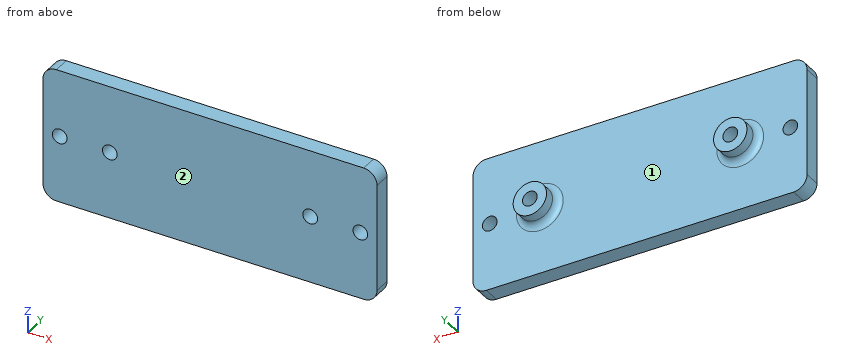
from build123d import *

# Parameters (mm, degrees)
BOSS_EXTRUDE1_DEPTH = 3.175
SKETCH2_R           = 3.175
BOSS_EXTRUDE2_DEPTH = 3.175
SKETCH3_R           = 1.397
CUT_EXTRUDE1_DEPTH  = 7.35
FILLET1_R           = 1.27
CUT_EXTRUDE2_REACH  = 5.175
SKETCH4_R           = 1.397


with BuildPart() as part:
    # Sketch1 → Boss-Extrude1 (new body)
    with BuildSketch(Plane(origin=(0, 0, 0), x_dir=(1, 0, 0), z_dir=(0, 1, 0))):
        with BuildLine():
            Line((-29.21, -12.7), (29.21, -12.7))
            ThreePointArc((29.21, -12.7), (31.006051224, -11.956051224), (31.75, -10.16))
            Line((31.75, -10.16), (31.75, 10.16))
            ThreePointArc((31.75, 10.16), (31.006051224, 11.956051224), (29.21, 12.7))
            Line((29.21, 12.7), (-29.21, 12.7))
            ThreePointArc((-29.21, 12.7), (-31.006051224, 11.956051224), (-31.75, 10.16))
            Line((-31.75, 10.16), (-31.75, -10.16))
            ThreePointArc((-31.75, -10.16), (-31.006051224, -11.956051224), (-29.21, -12.7))
        make_face()
    extrude(amount=BOSS_EXTRUDE1_DEPTH)

    # Sketch2 → Boss-Extrude2 (add)
    with BuildSketch(Plane(origin=(0, 3.175, 0), x_dir=(1, 0, 0), z_dir=(0, 1, 0))):
        with Locations((-19.05, 0)):
            Circle(SKETCH2_R)
        with Locations((19.05, 0)):
            Circle(SKETCH2_R)
    extrude(amount=BOSS_EXTRUDE2_DEPTH)

    # Sketch3 → Cut-Extrude1 (cut, through all)
    with BuildSketch(Plane(origin=(0, 6.35, 0), x_dir=(1, 0, 0), z_dir=(0, 1, 0))):
        with Locations((-19.05, 0)):
            Circle(SKETCH3_R)
        with Locations((19.05, 0)):
            Circle(SKETCH3_R)
    extrude(amount=-CUT_EXTRUDE1_DEPTH, mode=Mode.SUBTRACT)

    # Fillet1
    fillet1_edges = [part.edges().sort_by_distance(p)[0] for p in [
        (-22.225, 3.175, 0),
        (15.875, 3.175, 0),
    ]]
    fillet(fillet1_edges, radius=FILLET1_R)

    # Sketch4 → Cut-Extrude2 (cut, up to next)
    with BuildSketch(Plane(origin=(0, 3.175, 0), x_dir=(1, 0, 0), z_dir=(0, 1, 0)), mode=Mode.PRIVATE) as cut_extrude2_sk1:
        with Locations((-28.575, 0)):
            Circle(SKETCH4_R)
    cut_extrude2_tool1 = extrude(cut_extrude2_sk1.sketch, amount=-CUT_EXTRUDE2_REACH, mode=Mode.PRIVATE) & part.part
    add(cut_extrude2_tool1.solids().sort_by_distance((-28.575, 3.175, 0))[0], mode=Mode.SUBTRACT)
    # Sketch4 → Cut-Extrude2 (cut, up to next)
    with BuildSketch(Plane(origin=(0, 3.175, 0), x_dir=(1, 0, 0), z_dir=(0, 1, 0)), mode=Mode.PRIVATE) as cut_extrude2_sk2:
        with Locations((28.575, 0)):
            Circle(SKETCH4_R)
    cut_extrude2_tool2 = extrude(cut_extrude2_sk2.sketch, amount=-CUT_EXTRUDE2_REACH, mode=Mode.PRIVATE) & part.part
    add(cut_extrude2_tool2.solids().sort_by_distance((28.575, 3.175, 0))[0], mode=Mode.SUBTRACT)


solid = part.part
Build history of the part. All positions in model axes, mm. Face numbers are marked on the shaded views. Round coordinates to 2 decimals unless told otherwise and drop trailing zeros. Write each loop counter-clockwise with the first axis right and the second up, starting at its lowest first coordinate (ties: lowest second). Pieces come first, ordered by that corner, then holes. Notation, with made-up numbers: M 7,66 L 28,66 A26 cw 28,103 Z; hole C 39.5,27 d2. An arc over 180 degrees is marked long. Answer as a JSON object with one key per item and string values. Group by question number.
(1) Cut at C-C (y = 1.5). Give the cut face in (x, z) (3 decimals), and give its area (3 significant figures).
(2) Cut at A-A (x = 19.05). Give the cut face in (y, z) (3 decimals), and give its area (3 significant figures).
(3) Drill centre lines: L1, parallel to X at y = 2.05, z = 0; L2, parallel to X at y = 3.5, z = 0.75; L3, parallel to Y at x = 3, z = -11.5 (3 decimals). Where is each one in solid material? Low to high.
(4) Mould opens along X. For the marked faces 1 and 2 say: pulls with the +X half, pulls with the -X half, needs draft (parallel to the pull), parting line crosses it, or undercut.
(5) Cut at D-D (z = -6). Give the cut face in (x, y) (3 decimals), and give its area (3 significant figures).
(6) Flat gauge pins, fed straight in: pin 1 (3 mm diameter, centred on x = 3, z = 4, fed in from +Y) (3 decimals); pin 2 (1 mm diameter, centred on x = -21.5, y = 5, fed in from -Z). Where does each tip first touch, or does it go through?
(7) Cut at B-B (z = 0). Give the number of separate pieces and of enclosed holes in the cut face, and give its area (3 significant figures).
Responses:
{
 "1": {"outline": "M -31.75,-10.16 A2.54 ccw -29.21,-12.7 L 29.21,-12.7 A2.54 ccw 31.75,-10.16 L 31.75,10.16 A2.54 ccw 29.21,12.7 L -29.21,12.7 A2.54 ccw -31.75,10.16 Z; hole C -28.575,0 d2.794; hole C -19.05,0 d2.794; hole C 19.05,0 d2.794; hole C 28.575,0 d2.794", "area": "1,580 mm2"},
 "2": {"outline": "M 0,-12.7 L 3.175,-12.7 L 3.175,-4.445 A1.27 cw 4.445,-3.175 L 6.35,-3.175 L 6.35,-1.397 L 0,-1.397 Z; M 0,1.397 L 6.35,1.397 L 6.35,3.175 L 4.445,3.175 A1.27 cw 3.175,4.445 L 3.175,12.7 L 0,12.7 Z", "area": "83.8 mm2"},
 "3": {"L1": "x = -31.75 to -29.97, -27.18 to -20.45, -17.65 to 17.65, 20.45 to 27.18, 29.97 to 31.75", "L2": "x = -22.57 to -20.23, -17.87 to -15.53, 15.53 to 17.87, 20.23 to 22.57", "L3": "y = 0 to 3.175"},
 "4": {"face 1": "undercut", "face 2": "needs draft"},
 "5": {"outline": "M -31.75,0 L 31.75,0 L 31.75,3.175 L -31.75,3.175 Z", "area": "202 mm2"},
 "6": {"pin 1": "stops at y = 3.175", "pin 2": "stops at z = -2.51"},
 "7": {"separate pieces": "5", "enclosed holes": "0", "area": "190 mm2"}
}
